from build123d import *

# Parameters (mm, degrees)
RESSALTO_EXTRUS_O1_DEPTH = 2.5
FILETE1_R                = 0.1


with BuildPart() as part:
    # Esboço1 → Ressalto-extrusão1 (new body)
    with BuildSketch(Plane.XY):
        with BuildLine():
            Line((60.523872434, -95.459023636), (60.523872434, -100.759023636))
            Line((60.523872434, -100.759023636), (69.023872434, -100.759023636))
            Line((69.023872434, -100.759023636), (69.023872434, -96.859023636))
            Line((69.023872434, -96.859023636), (71.523872434, -96.859023636))
            Line((71.523872434, -96.859023636), (71.523872434, -100.759023636))
            Line((71.523872434, -100.759023636), (151.523872434, -100.759023636))
            Line((151.523872434, -100.759023636), (151.523872434, -96.859023636))
            Line((151.523872434, -96.859023636), (154.023872434, -96.859023636))
            Line((154.023872434, -96.859023636), (154.023872434, -100.759023636))
            Line((154.023872434, -100.759023636), (158.523872434, -100.759023636))
            Line((158.523872434, -100.759023636), (158.523872434, -95.459023636))
            ThreePointArc((158.523872434, -95.459023636), (156.473619903, -90.509276168), (151.523872434, -88.459023636))
            Line((151.523872434, -88.459023636), (67.523872434, -88.459023636))
            ThreePointArc((67.523872434, -88.459023636), (62.574124966, -90.509276168), (60.523872434, -95.459023636))
        make_face()
    extrude(amount=RESSALTO_EXTRUS_O1_DEPTH)

    # Filete1
    filete1_edges = [part.edges().sort_by_distance(p)[0] for p in [
        (64.773872434, -100.759023636, 2.5),
        (109.523872434, -88.459023636, 0),
        (156.473619903, -90.509276168, 0),
        (158.523872434, -98.109023636, 0),
        (156.273872434, -100.759023636, 0),
        (154.023872434, -98.809023636, 0),
        (152.773872434, -96.859023636, 0),
        (69.023872434, -98.809023636, 2.5),
        (151.523872434, -98.809023636, 0),
        (111.523872434, -100.759023636, 0),
        (71.523872434, -98.809023636, 0),
        (70.273872434, -96.859023636, 0),
        (69.023872434, -98.809023636, 0),
        (64.773872434, -100.759023636, 0),
        (60.523872434, -98.109023636, 0),
        (62.574124966, -90.509276168, 0),
        (70.273872434, -96.859023636, 2.5),
        (71.523872434, -98.809023636, 2.5),
        (158.523872434, -100.759023636, 1.25),
        (154.023872434, -100.759023636, 1.25),
        (154.023872434, -96.859023636, 1.25),
        (151.523872434, -96.859023636, 1.25),
        (151.523872434, -100.759023636, 1.25),
        (71.523872434, -100.759023636, 1.25),
        (71.523872434, -96.859023636, 1.25),
        (69.023872434, -96.859023636, 1.25),
        (69.023872434, -100.759023636, 1.25),
        (60.523872434, -100.759023636, 1.25),
        (111.523872434, -100.759023636, 2.5),
        (151.523872434, -98.809023636, 2.5),
        (152.773872434, -96.859023636, 2.5),
        (154.023872434, -98.809023636, 2.5),
        (156.273872434, -100.759023636, 2.5),
        (158.523872434, -98.109023636, 2.5),
        (62.574124966, -90.509276168, 2.5),
        (156.473619903, -90.509276168, 2.5),
        (109.523872434, -88.459023636, 2.5),
        (60.523872434, -98.109023636, 2.5),
    ]]
    fillet(filete1_edges, radius=FILETE1_R)


solid = part.part
For this review, take the finished solid that the model builds, in its own axes (mm). A direction names the side the tool comes from. Round coordinates to 2 decimals unless told otherwise and drop trailing zeros. Order: outer loops, then holes, each group sorted by start corner. A loop starts at its lowest first (then second) coordinate and runs counter-clockwise, first axis right, second up. Notation, with made-up numbers: (28, 46) -> (38, 46) arc R9 cw to (38, 52) -> close; hole circle Ø8 at (38.25, -1.75). An arc over 180 degrees is marked (long way). Write item = value, one per line. Start each with the question number.
1) To check wall thickness, follow line 1 (X direction, y = -98.25, z = 1.25); line 2 (Y direction, x = 70.5, z = 0.35); line 3 (Y direction, x = 67, z = 1.8). State the ranges of each line that lie inside material, in increasing order. Write a range as from..to.
2) Take a section at A-A on y = -99.5. State the section outline as (x, z) points, plus the area to 3 significant figures.
3) Insertion check: pin 1 (0.7 mm diameter, centred on x = 70, z = 1, fed in from -Y). The pin has a flat end and moves straight along its axis. Give the tip position at first contact, or say it passes through.
4) Tool access review of faces 5 (the face through (156.528, -90.564, 1.234)), 6 (the face through (70, -96.859, 1)): name each direction out of +Z, -Z, +X, -X, +Y, -Y from which nothing blocks a thin tool from reaching the whole face with its end or side.
5) The part is to be moulded in two halves that separate along X. For faces 1 (the face through (62.629, -90.455, 1.234)), 2 (the face through (151.524, -99, 1)), 3 (the face through (153, -96.859, 1)), 4 (the face through (158.524, -98, 1)), say which applies: +X half, -X half, draft (parallel to the pull), parting line (faces both ways), or undercut.
6) Take a section at B-B on z = 2. State the section outline as (x, y) points, plus the area to 3 significant figures.
Verdict:
q1.line_1 = 60.52..69.02, 71.52..151.52, 154.02..158.52
q1.line_2 = -96.86..-88.46
q1.line_3 = -100.76..-88.48
q2.outline = (60.52, 0.1) arc R0.1 ccw to (60.62, 0) -> (68.92, 0) arc R0.1 ccw to (69.02, 0.1) -> (69.02, 2.4) arc R0.1 ccw to (68.92, 2.5) -> (60.62, 2.5) arc R0.1 ccw to (60.52, 2.4) -> close; (71.52, 0.1) arc R0.1 ccw to (71.62, 0) -> (151.42, 0) arc R0.1 ccw to (151.52, 0.1) -> (151.52, 2.4) arc R0.1 ccw to (151.42, 2.5) -> (71.62, 2.5) arc R0.1 ccw to (71.52, 2.4) -> close; (154.02, 0.1) arc R0.1 ccw to (154.12, 0) -> (158.42, 0) arc R0.1 ccw to (158.52, 0.1) -> (158.52, 2.4) arc R0.1 ccw to (158.42, 2.5) -> (154.12, 2.5) arc R0.1 ccw to (154.02, 2.4) -> close
q2.area = 232 mm2
q3.pin_1 = -96.86
q4.face_5 = +Z, -Z, +X, +Y
q4.face_6 = +Z, -Z, -Y
q5.face_1 = -X half
q5.face_2 = undercut
q5.face_3 = undercut
q5.face_4 = +X half
q6.outline = (60.52, -100.66) arc R0.1 ccw to (60.62, -100.76) -> (68.92, -100.76) arc R0.1 ccw to (69.02, -100.66) -> (69.02, -96.96) arc R0.1 cw to (69.12, -96.86) -> (71.42, -96.86) arc R0.1 cw to (71.52, -96.96) -> (71.52, -100.66) arc R0.1 ccw to (71.62, -100.76) -> (151.42, -100.76) arc R0.1 ccw to (151.52, -100.66) -> (151.52, -96.96) arc R0.1 cw to (151.62, -96.86) -> (153.92, -96.86) arc R0.1 cw to (154.02, -96.96) -> (154.02, -100.66) arc R0.1 ccw to (154.12, -100.76) -> (158.42, -100.76) arc R0.1 ccw to (158.52, -100.66) -> (158.52, -95.46) arc R7 ccw to (151.52, -88.46) -> (67.52, -88.46) arc R7 ccw to (60.52, -95.46) -> close
q6.area = 1,160 mm2
